CAD build for the part. Positions are in the model's coordinates, mm. A direction names the side the tool comes from. Coordinates: 2 decimals unless noted, no trailing zeros. Loops run counter-clockwise (first coordinate to the right, second up) from the corner with the lowest first, then second, coordinate; pieces in that order, holes last. Notation, with made-up numbers: (25, 41) -> (68, 41) arc R17 cw to (68, 74) -> close; hole circle Ø4 at (-1, 51). An arc over 180 degrees is marked (long way). Answer as a JSON object with one key per item and string values. Group by question number.
from build123d import *

# Parameters (mm, degrees)
F0_R     = 1.5875
F0_W     = 52.3748
F0_H     = 52.3748
F1_DEPTH = 5.207


with BuildPart() as f1:
    # F0 (on Front) → F1 (new body)
    with BuildSketch(Plane.XZ):
        with BuildLine():
            Line((-29.9466, -33.7566), (29.9466, -33.7566))
            ThreePointArc((29.9466, -33.7566), (32.640677, -32.640677), (33.7566, -29.9466))
            Line((33.7566, -29.9466), (33.7566, 29.9466))
            ThreePointArc((33.7566, 29.9466), (32.640677, 32.640677), (29.9466, 33.7566))
            Line((29.9466, 33.7566), (-29.9466, 33.7566))
            ThreePointArc((-29.9466, 33.7566), (-32.640677, 32.640677), (-33.7566, 29.9466))
            Line((-33.7566, 29.9466), (-33.7566, -29.9466))
            ThreePointArc((-33.7566, -29.9466), (-32.640677, -32.640677), (-29.9466, -33.7566))
        make_face()
        with Locations((-29.972, 0)):
            Circle(F0_R, mode=Mode.SUBTRACT)
        Rectangle(F0_W, F0_H, mode=Mode.SUBTRACT)
        with Locations((29.972, 0)):
            Circle(F0_R, mode=Mode.SUBTRACT)
    extrude(amount=F1_DEPTH)


solid = f1.part
Item 1: Band-saw the part on A-A, the plane z = -7. List the corners of the cut face in (x, y).
Item 2: Pull direction X, two halves, no side cores. Call faces 1 (the flat face through (-33.757, -3, 0)), 2 (the cylindrical face through (31.486, -2.567, 0.477)), 3 (the flat face through (0, -3, -33.757)): +X half, -X half, draft (parallel to the pull), parting line (faces both ways), or undercut.
Item 3: Band-saw the part on C-C, the plane z = 0. List the corners of the cut face in (x, y), and give its area (3 significant figures).
Item 4: Band-saw the part on D-D, the plane y = -4.1. List the corners of the cut face in (x, z) (1 decimal).
Item 5: 3-axis set-ups, long thin cutter, end or side, ignore diameter. For faces 4 (the flat face through (-26.187, -3, 0)), 5 (the cylindrical face through (32.67, -2.57, 32.61)): which of +Z, -Z, +X, -X, +Y, -Y reach the whole face in a straight line?
Item 6: Drill centre line: L1, parallel to X at y = -3.2, z = 11.5. Where is it in solid material? Low to high.
Item 7: Flat gauge pin, fed straight in: P1, Ø2, axis at x = -25, z = -23, coming from the -Y side. Where does the tip first touch, or does it go through?
Item 8: Band-saw the part on B-B, the plane x = 23. List the corners of the cut face in (y, z).
Reply:
{
 "1": {"outline": "(-33.76, -5.21) -> (-26.19, -5.21) -> (-26.19, 0) -> (-33.76, 0) -> close; (26.19, -5.21) -> (33.76, -5.21) -> (33.76, 0) -> (26.19, 0) -> close"},
 "2": {"face 1": "-X half", "face 2": "undercut", "face 3": "draft"},
 "3": {"outline": "(-33.76, -5.21) -> (-31.56, -5.21) -> (-31.56, 0) -> (-33.76, 0) -> close; (-28.38, -5.21) -> (-26.19, -5.21) -> (-26.19, 0) -> (-28.38, 0) -> close; (26.19, -5.21) -> (28.38, -5.21) -> (28.38, 0) -> (26.19, 0) -> close; (31.56, -5.21) -> (33.76, -5.21) -> (33.76, 0) -> (31.56, 0) -> close", "area": "45.8 mm²"},
 "4": {"outline": "(-33.8, -29.9) arc R3.8 ccw to (-29.9, -33.8) -> (29.9, -33.8) arc R3.8 ccw to (33.8, -29.9) -> (33.8, 29.9) arc R3.8 ccw to (29.9, 33.8) -> (-29.9, 33.8) arc R3.8 ccw to (-33.8, 29.9) -> close; hole circle Ø3.2 at (-30, 0); hole (-26.2, -26.2) -> (26.2, -26.2) -> (26.2, 26.2) -> (-26.2, 26.2) -> close; hole circle Ø3.2 at (30, 0)"},
 "5": {"face 4": "+Y, -Y", "face 5": "+Z, +X, +Y, -Y"},
 "6": {"L1": "-33.76 to -26.19, 26.19 to 33.76"},
 "7": {"P1": "through"},
 "8": {"outline": "(-5.21, -33.76) -> (0, -33.76) -> (0, -26.19) -> (-5.21, -26.19) -> close; (-5.21, 26.19) -> (0, 26.19) -> (0, 33.76) -> (-5.21, 33.76) -> close"}
}
